Source: CAD feature listing. Evaluate the final solid. Frame: model axes, mm. A direction names the side the tool comes from. Coordinates: 2 decimals unless noted, no trailing zeros. Write each loop counter-clockwise with the first axis right and the second up, starting at its lowest first coordinate (ties: lowest second). Pieces come first, ordered by that corner, then holes. Notation, with made-up numbers: (-21, -29.75) - (3, -29.75) arc R13 ccw to (3, -14.75) - close; hole circle Ø2 at (43.25, 21). An arc over 180 degrees is marked (long way). One line per question, with ' | ' between items.
from build123d import *

# Parameters (mm, degrees)
BOSS_EXTRUDE4_DEPTH = 5
SKETCH6_W           = 70
SKETCH6_H           = 70
BOSS_EXTRUDE5_DEPTH = 5
SKETCH8_R           = 3
CUT_EXTRUDE1_DEPTH  = 2
FILLET1_R           = 10
CUT_EXTRUDE2_DEPTH  = 145.654761415
CHAMFER1_SIZE       = 1.25


with BuildPart() as part:
    # Sketch5 → Boss-Extrude4 (new body)
    with BuildSketch(Plane(origin=(0, 0, 0), x_dir=(1, 0, 0), z_dir=(0, 1, 0))):
        with BuildLine():
            Line((-22.5, -32.5), (22.5, -32.5))
            ThreePointArc((22.5, -32.5), (29.571067812, -29.571067812), (32.5, -22.5))
            Line((32.5, -22.5), (32.5, 22.5))
            ThreePointArc((32.5, 22.5), (29.571067812, 29.571067812), (22.5, 32.5))
            Line((22.5, 32.5), (-22.5, 32.5))
            ThreePointArc((-22.5, 32.5), (-29.571067812, 29.571067812), (-32.5, 22.5))
            Line((-32.5, 22.5), (-32.5, -22.5))
            ThreePointArc((-32.5, -22.5), (-29.571067812, -29.571067812), (-22.5, -32.5))
        make_face()
    extrude(amount=BOSS_EXTRUDE4_DEPTH)

    # Sketch6 → Boss-Extrude5 (add)
    with BuildSketch(Plane(origin=(0, 5, 0), x_dir=(1, 0, 0), z_dir=(0, 1, 0))):
        Rectangle(SKETCH6_W, SKETCH6_H)
    extrude(amount=BOSS_EXTRUDE5_DEPTH)

    # Sketch8 → Cut-Extrude1 (cut)
    with BuildSketch(Plane.XZ):
        with Locations(Location((26.037533906, -26.035533906, 0), (0, 0, 270))):
            Circle(SKETCH8_R)
        with Locations(Location((26.036533906, 26.036533906, 0), (0, 0, 270))):
            Circle(SKETCH8_R)
        with BuildLine():
            ThreePointArc((-23.035533906, 26.035533906), (-24.887483609, 28.807172503), (-28.156854249, 28.156854249))
            Line((-28.156854249, 28.156854249), (-23.914213562, 23.914213562))
            ThreePointArc((-23.914213562, 23.914213562), (-23.263895308, 24.887483609), (-23.035533906, 26.035533906))
        make_face()
        with BuildLine():
            Line((-23.914213562, 23.914213562), (-28.156854249, 28.156854249))
            ThreePointArc((-28.156854249, 28.156854249), (-28.156854249, 23.914213562), (-23.914213562, 23.914213562))
        make_face()
        with Locations(Location((-26.034533906, -26.036533906, 0), (0, 0, 270))):
            Circle(SKETCH8_R)
    extrude(amount=-CUT_EXTRUDE1_DEPTH, mode=Mode.SUBTRACT)

    # Mirror1: part across plane


with BuildPart() as part_1:
    add(part.part)
    add(part.part.mirror(Plane(origin=(-35, 10, -35), x_dir=(0, 0, 1), z_dir=(1, 0, 0))))

    # Fillet1
    fillet1_edges = [part_1.edges().sort_by_distance(p)[0] for p in [
        (35, 7.5, 35),
        (35, 7.5, -35),
        (-105, 7.5, 35),
        (-105, 7.5, -35),
    ]]
    fillet(fillet1_edges, radius=FILLET1_R)

    # Sketch9 → Cut-Extrude2 (cut, through all)
    with BuildSketch(Plane(origin=(35, 0, 0), x_dir=(0, 0, -1), z_dir=(1, 0, 0))):
        Polygon((17.878679656, 10), (22.121320344, 10), (26.060660172, 6.060660172), (27.121320344, 5), (22.878679656, 5), (18.939339828, 8.939339828), align=None)
    extrude(amount=-CUT_EXTRUDE2_DEPTH, mode=Mode.SUBTRACT)

    # Chamfer1
    chamfer1_edges = [part_1.edges().sort_by_distance(p)[0] for p in [
        (-105, 10, 3.560660172),
        (-35, 10, -35),
        (-35, 10, 35),
        (35, 10, 3.560660172),
        (32.071067812, 10, -32.071067812),
        (32.071067812, 10, 32.071067812),
        (-102.071067812, 10, 32.071067812),
        (-102.071067812, 10, -32.071067812),
        (-105, 10, -23.560660172),
        (35, 10, -23.560660172),
    ]]
    chamfer(chamfer1_edges, length=CHAMFER1_SIZE)


solid = part_1.part
Item 1: Cut plane A-A on z = 12.5. Return loops of the section in (x, y), and give its area (3 significant figures).
Check sheet entries:
outline: (-105, 5) - (-102.5, 5) - (-102.5, 0) - (-37.5, 0) - (-37.5, 5) - (-32.5, 5) - (-32.5, 0) - (32.5, 0) - (32.5, 5) - (35, 5) - (35, 8.75) - (33.75, 10) - (-103.75, 10) - (-105, 8.75) - close | area: 1,350 mm²
Item 2: Cut plane B-B on x = -19. Return loops of the section in (y, z), and give its area (3 significant figures).
Check sheet entries:
outline: (0, -32.5) - (5, -32.5) - (5, -35) - (8.75, -35) - (10, -33.75) - (10, -22.12) - (5, -27.12) - (5, -22.88) - (10, -17.88) - (10, 33.75) - (8.75, 35) - (5, 35) - (5, 32.5) - (0, 32.5) - close | area: 652 mm²
Item 3: Mould query, pull axis Y, two halves, no side actions, for faces 1 (the face through (-34, 10, 8)), 2 (the face through (-96, 2, 26)), 3 (the face through (-24.007, 0.986, -23.825)), 4 (the face through (-34.02, 7.46, -24.66)). Classes: pulls with the +Y half, pulls with the -Y half, needs draft (parallel to the pull), parting line crosses it, or undercut.
Check sheet entries:
face 1: pulls with the +Y half | face 2: pulls with the -Y half | face 3: needs draft | face 4: undercut
Item 4: Pin query (flat end, axial travel): pin 1 Ø2.5 at (y, z) = (3.5, 5.5) entering from -X; pin 2 Ø3 at (x, z) = (-43, -25.5) entering from -Y; pin 3 Ø1.5 at (x, y) = (6, 3) entering from +Z. Return the tip coordinate at first contact, or that it passes through.
Check sheet entries:
pin 1: x = -102.5 | pin 2: y = 2 | pin 3: z = 32.5
Item 5: Ray query, line 1 along X through (y, z) = (0.5, -5); line 2 along Z through (x, y) = (14.5, 2.5); line 3 along Z through (x, y) = (-86, 5.25). Return the intervals inside material, ascending. Write a range as [from, to].
Check sheet entries:
line 1: [-102.5, -37.5], [-32.5, 32.5] | line 2: [-32.5, 32.5] | line 3: [-35, -26.87], [-22.63, 35]
Item 6: Access query for faces 5 (the face through (-96, 2, -26)), 6 (the face through (-70, 2, 32.5)), 7 (the face through (32.5, 2, 0)), 8 (the face through (-37.5, 2, 0)). Directions: +Z, -Z, +X, -X, +Y, -Y. A direction counts if a zero-diameter tool reaches every point of the face in a straight line with its end or side. Return the directions, or none.
Check sheet entries:
face 5: -Y | face 6: +Z, +X, -X, -Y | face 7: +Z, -Z, +X, -Y | face 8: +Z, -Z, -Y
